The model under review builds one solid part; all positions refer to its coordinate system, in mm. Face numbers are marked on the shaded views. A direction names the side the tool comes from. Round coordinates to 2 decimals unless told otherwise and drop trailing zeros. Order: outer loops, then holes, each group sorted by start corner. A loop starts at its lowest first (then second) coordinate and runs counter-clockwise, first axis right, second up.
1) Machinability: for the marked faces 1, 2, 3 and 4, which of the approach directions +Z, -Z, +X, -X, +Y, -Y give a long, thin tool a straight path to every point of the face, cutting with its end or side? Answer none if there is none.
2) Clearance check with flat-ended pins moving along their axes: P1, Ø1.2, axis at y = 54.5, z = 1.5, coming from the -X side; P2, Ø0.7, axis at x = 0, z = 1.5, coming from the -Y side; P3, Ø3, axis at y = 4, z = 3.5, coming from the +X side. State where each tip first meets the part, or that it passes through.
3) Consider section C-C (y = 29). Give the boundary of the cut face in (x, z).
4) Consider section A-A (x = 22). Give the boundary of the cut face in (y, z), then the cut area to 3 significant figures.
5) To check wall thickness, follow L1, parallel to Y at x = 26, z = 1.35; L2, parallel to Y at x = -8, z = 4.3; L3, parallel to Y at x = 27, z = 4.45. State the ranges of each line that lie inside material, in increasing order.
6) Consider section D-D (x = 8). Give the boundary of the cut face in (y, z).
7) Mouldability with a two-part tool opening along Y and no side actions: class the marked faces 5, 6 and 7 as pulls with the +Y half, pulls with the -Y half, needs draft (parallel to the pull), parting line crosses it, or undercut.
from build123d import *

# Parameters (mm, degrees)
BOSS_EXTRUDE1_DEPTH = 5.08
BOSS_EXTRUDE2_DEPTH = 5.08


with BuildPart() as part:
    # Sketch1 → Boss-Extrude1 (new body)
    with BuildSketch(Plane.XY):
        with BuildLine():
            Line((-9.251487929, 55.88), (0.551476187, 55.88))
            ThreePointArc((0.551476187, 55.88), (0.910686432, 55.731210245), (1.059476187, 55.372))
            Line((1.059476187, 55.372), (1.059476187, 53.848))
            ThreePointArc((1.059476187, 53.848), (0.910686432, 53.488789755), (0.551476187, 53.34))
            Line((0.551476187, 53.34), (-0.762, 53.34))
            ThreePointArc((-0.762, 53.34), (-1.121210245, 53.191210245), (-1.27, 52.832))
            Line((-1.27, 52.832), (-1.27, 51.308))
            ThreePointArc((-1.27, 51.308), (-1.121210245, 50.948789755), (-0.762, 50.8))
            Line((-0.762, 50.8), (1.059476187, 50.8))
            ThreePointArc((1.059476187, 50.8), (3.071209903, 49.810653879), (3.515777519, 47.613328704))
            Line((3.515777519, 47.613328704), (-15.208009334, -23.506671296))
            ThreePointArc((-15.208009334, -23.506671296), (-16.113656787, -24.871733717), (-17.664310667, -25.4))
            Line((-17.664310667, -25.4), (-19.05, -25.4))
            Line((-19.05, -25.4), (-19.05, 48.26))
            ThreePointArc((-19.05, 48.26), (-18.306051224, 50.056051224), (-16.51, 50.8))
            Line((-16.51, 50.8), (-4.092493287, 50.8))
            ThreePointArc((-4.092493287, 50.8), (-3.733283042, 50.948789755), (-3.584493287, 51.308))
            Line((-3.584493287, 51.308), (-3.584493287, 52.832))
            ThreePointArc((-3.584493287, 52.832), (-3.733283042, 53.191210245), (-4.092493287, 53.34))
            Line((-4.092493287, 53.34), (-9.251487929, 53.34))
            ThreePointArc((-9.251487929, 53.34), (-9.610698174, 53.488789755), (-9.759487929, 53.848))
            Line((-9.759487929, 53.848), (-9.759487929, 55.372))
            ThreePointArc((-9.759487929, 55.372), (-9.610698174, 55.731210245), (-9.251487929, 55.88))
        make_face()
    extrude(amount=BOSS_EXTRUDE1_DEPTH)

    # Sketch3 → Boss-Extrude2 (add)
    with BuildSketch(Plane.XY.offset(5.08)):
        with BuildLine():
            Line((29.21, 10.16), (0, 10.16))
            Line((0, 10.16), (-3.049315827, 10.16))
            ThreePointArc((-3.049315827, 10.16), (-5.061049543, 11.149346121), (-5.505617159, 13.346671296))
            Line((-5.505617159, 13.346671296), (-9.703476753, -2.598381736))
            ThreePointArc((-9.703476753, -2.598381736), (-6.986534394, 1.496805525), (-2.334572756, 3.081604376))
            Line((-2.334572756, 3.081604376), (26.819356948, 3.081604376))
            Line((26.819356948, 3.081604376), (26.819356948, 5.616399787))
            Line((26.819356948, 5.616399787), (18.639798787, 5.616399787))
            Line((18.639798787, 5.616399787), (18.639798787, 7.62))
            Line((18.639798787, 7.62), (29.21, 7.62))
            Line((29.21, 7.62), (29.21, 10.16))
        make_face()
    extrude(amount=-BOSS_EXTRUDE2_DEPTH)


solid = part.part
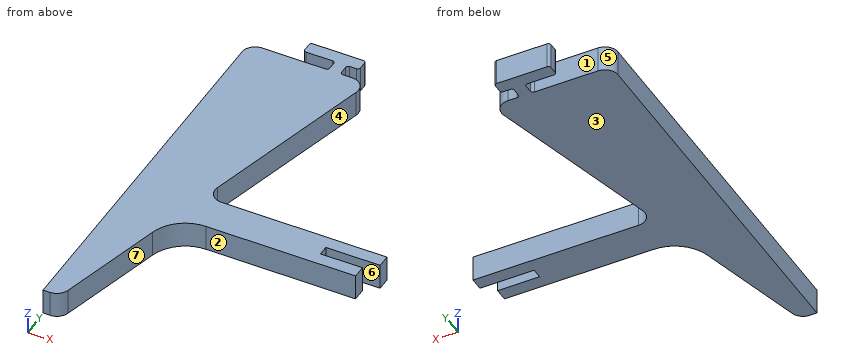
Answer below:
1. face 1: +Z, -Z, -X
1. face 2: +Z, -Z, +X, -Y
1. face 3: -Z, +X, -X, +Y, -Y
1. face 4: +Z, -Z, +X
2. P1: stops at x = -9.76
2. P2: stops at y = 3.08
2. P3: stops at x = 26.82
3. outline: (-19.05, 0) - (-1.38, 0) - (-1.38, 5.08) - (-19.05, 5.08) - close
4. outline: (3.08, 0) - (5.62, 0) - (5.62, 5.08) - (3.08, 5.08) - close; (7.62, 0) - (10.16, 0) - (10.16, 5.08) - (7.62, 5.08) - close
4. area: 25.8 mm2
5. L1: y = 3.08 to 5.62, 7.62 to 10.16
5. L2: y = 0.56 to 50.8, 53.34 to 55.88
5. L3: y = 7.62 to 10.16
6. outline: (3.08, 0) - (10.16, 0) - (10.16, 5.08) - (3.08, 5.08) - close
7. face 5: pulls with the +Y half
7. face 6: undercut
7. face 7: pulls with the -Y half
